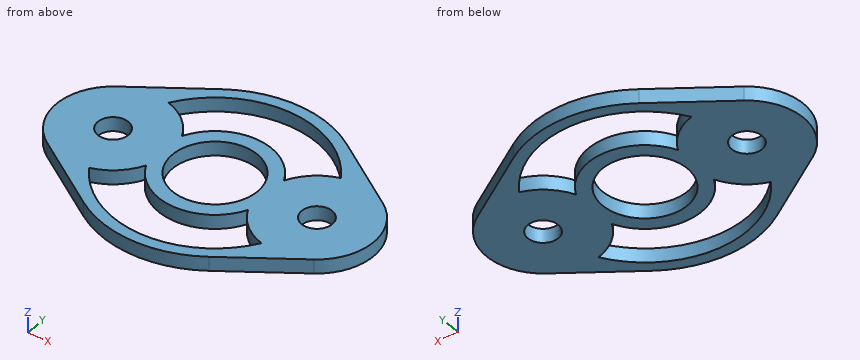
from build123d import *

# Parameters (mm, degrees)
F0_R     = 3.429
F0_R_2   = 9.525
F1_DEPTH = 3.175


with BuildPart() as f1:
    # F0 (on Top) → F1 (new body)
    with BuildSketch(Plane.XY):
        with BuildLine():
            Line((8.748889, 21.119577), (-7.055556, 10.559789))
            ThreePointArc((-7.055556, 10.559789), (-12.7, 0), (-7.055556, -10.559789))
            Line((-7.055556, -10.559789), (8.748889, -21.119577))
            ThreePointArc((8.748889, -21.119577), (22.86, -25.4), (36.971111, -21.119577))
            Line((36.971111, -21.119577), (52.775556, -10.559789))
            ThreePointArc((52.775556, -10.559789), (58.42, 0), (52.775556, 10.559789))
            Line((52.775556, 10.559789), (36.971111, 21.119577))
            ThreePointArc((36.971111, 21.119577), (22.86, 25.4), (8.748889, 21.119577))
        make_face()
        with BuildLine():
            ThreePointArc((42.192222, -12.200196), (22.86, -22.86), (3.527778, -12.200196))
            ThreePointArc((3.527778, -12.200196), (8.187632, -9.708382), (11.43, -5.535802))
            ThreePointArc((11.43, -5.535802), (22.86, -12.7), (34.29, -5.535802))
            ThreePointArc((34.29, -5.535802), (37.532368, -9.708382), (42.192222, -12.200196))
        make_face(mode=Mode.SUBTRACT)
        Circle(F0_R, mode=Mode.SUBTRACT)
        with Locations((22.86, 0)):
            Circle(F0_R_2, mode=Mode.SUBTRACT)
        with Locations((45.72, 0)):
            Circle(F0_R, mode=Mode.SUBTRACT)
        with BuildLine():
            ThreePointArc((42.192222, 12.200196), (37.532368, 9.708382), (34.29, 5.535802))
            ThreePointArc((34.29, 5.535802), (22.86, 12.7), (11.43, 5.535802))
            ThreePointArc((11.43, 5.535802), (8.187632, 9.708382), (3.527778, 12.200196))
            ThreePointArc((3.527778, 12.200196), (22.86, 22.86), (42.192222, 12.200196))
        make_face(mode=Mode.SUBTRACT)
    extrude(amount=F1_DEPTH)


solid = f1.part
CAD build for the part. Positions are in the model's coordinates, mm. Give positions to 0.01 mm unless a question says otherwise; leave off trailing zeros. Loops run counter-clockwise (first coordinate to the right, second up) from the corner with the lowest first, then second, coordinate; pieces in that order, holes last. Notation, with made-up numbers: M 24.5,60.5 L 32.5,60.5 A4 ccw 32.5,66.5 Z; hole C 49,-14 d11. An arc over 180 degrees is marked long. One line per question, with ' | ' between items. Start each with the question number.
1. Flat gauge pins, fed straight in: pin 1 (1.5 mm diameter, centred on x = 49, z = 1, fed in from +Y); pin 2 (1.5 mm diameter, centred on x = 36.5, z = 2.5, fed in from -Y); pin 3 (1 mm diameter, centred on y = -17.5, z = 1.5, fed in from -X). Where does each tip first touch, or does it go through?
2. Saw through at A-A on z = 0.5. Give the cut face in (x, y) (3 decimals).
3. Probe L1, parallel to X at y = -0.5, z = 2.7; L2, parallel to Y at x = 33.5, z = 0.6; L3, parallel to Y at x = 36, z = 2.15. List the from-to ranges inside material, lowest first. Write a range as from..to.
4. Saw through at B-B on y = 0. Give the cut face in (x, z) (3 decimals).
5. Saw through at D-D on x = 45.72. Give the cut face in (y, z) (3 decimals).
6. Saw through at C-C on x = 22.86. Give the cut face in (y, z) (3 decimals), plus the area to 3 significant figures.
Result sheet:
1) pin 1: stops at y = 13.58 | pin 2: stops at y = -21.89 | pin 3: stops at x = 2.58
2) outline: M -7.056,-10.56 L 8.749,-21.12 A25.4 ccw 36.971,-21.12 L 52.776,-10.56 A12.7 ccw 52.776,10.56 L 36.971,21.12 A25.4 ccw 8.749,21.12 L -7.056,10.56 A12.7 ccw Z; hole C 0,0 d6.858; hole M 3.528,-12.2 A22.86 ccw 42.192,-12.2 A12.7 cw 34.29,-5.536 A12.7 cw 11.43,-5.536 A12.7 cw Z; hole M 3.528,12.2 A12.7 cw 11.43,5.536 A12.7 cw 34.29,5.536 A12.7 cw 42.192,12.2 A22.86 ccw Z; hole C 22.86,0 d19.05; hole C 45.72,0 d6.858
3) L1: x = -12.69..-3.39, 3.39..13.35, 32.37..42.33, 49.11..58.41 | L2: y = -23.06..-20.23, -6.93..6.93, 20.23..23.06 | L3: y = -21.74..-18.71, -8.17..8.17, 18.71..21.74
4) outline: M -12.7,0 L -3.429,0 L -3.429,3.175 L -12.7,3.175 Z; M 3.429,0 L 13.335,0 L 13.335,3.175 L 3.429,3.175 Z; M 32.385,0 L 42.291,0 L 42.291,3.175 L 32.385,3.175 Z; M 49.149,0 L 58.42,0 L 58.42,3.175 L 49.149,3.175 Z
5) outline: M -15.274,0 L -3.429,0 L -3.429,3.175 L -15.274,3.175 Z; M 3.429,0 L 15.274,0 L 15.274,3.175 L 3.429,3.175 Z
6) outline: M -25.4,0 L -22.86,0 L -22.86,3.175 L -25.4,3.175 Z; M -12.7,0 L -9.525,0 L -9.525,3.175 L -12.7,3.175 Z; M 9.525,0 L 12.7,0 L 12.7,3.175 L 9.525,3.175 Z; M 22.86,0 L 25.4,0 L 25.4,3.175 L 22.86,3.175 Z | area: 36.3 mm^2
